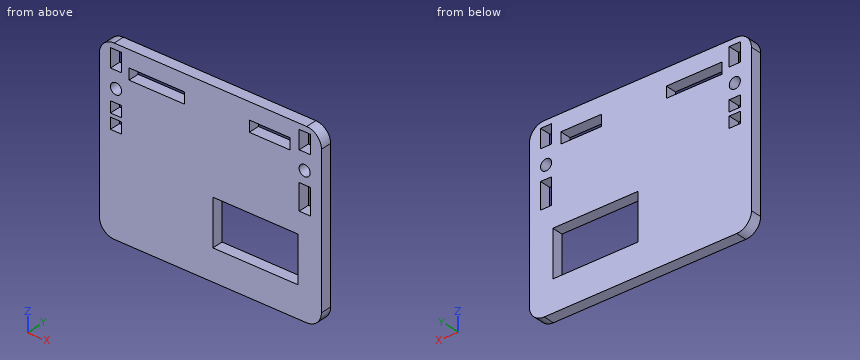
```python
from build123d import *

# Parameters (mm, degrees)
CROQUIS1_R                 = 1.5
CROQUIS1_W                 = 15
CROQUIS1_H                 = 3
CROQUIS1_W_2               = 3.003677296
CROQUIS1_H_2               = 7.000000001
CROQUIS1_W_3               = 23
CROQUIS1_H_3               = 12.400000001
SALIENTE_EXTRUIR1_DEPTH    = 3
S_LIDO_MOVER_COPIAR2_ANGLE = 90


with BuildPart() as part:
    # Croquis1 → Saliente-Extruir1 (new body)
    with BuildSketch(Plane(origin=(0, 0, 0), x_dir=(-1, 0, 0), z_dir=(0, 0, 1))):
        with BuildLine():
            Line((41781.908830987, 309.199124202), (41833.908830987, 309.199124202))
            ThreePointArc((41833.908830987, 309.199124202), (41836.737258112, 310.370697077), (41837.908830987, 313.199124202))
            Line((41837.908830987, 313.199124202), (41837.908830987, 353.199124202))
            ThreePointArc((41837.908830987, 353.199124202), (41836.737258112, 356.027551327), (41833.908830987, 357.199124202))
            Line((41833.908830987, 357.199124202), (41781.908830987, 357.199124202))
            ThreePointArc((41781.908830987, 357.199124202), (41779.080403863, 356.027551327), (41777.908830987, 353.199124202))
            Line((41777.908830987, 353.199124202), (41777.908830987, 313.199124202))
            ThreePointArc((41777.908830987, 313.199124202), (41779.080403863, 310.370697077), (41781.908830987, 309.199124202))
        make_face()
        with Locations(Location((41833.408830987, 320.199124198, 0), (0, 0, 180))):
            Circle(CROQUIS1_R, mode=Mode.SUBTRACT)
        with Locations(Location((41782.429915347, 320.197748539, 0), (0, 0, 180))):
            Circle(CROQUIS1_R, mode=Mode.SUBTRACT)
        Polygon((41786.408830987, 313.699124203), (41796.408830987, 313.699124203), (41797.408830987, 313.699124203), (41797.408830987, 316.699124203), (41796.408830987, 316.699124203), (41786.408830987, 316.699124203), align=None, mode=Mode.SUBTRACT)
        Polygon((41780.927290538, 315.695638799), (41783.429912384, 315.695638799), (41783.927165547, 315.695638799), (41783.929915347, 310.699124202), (41780.929915347, 310.699124202), align=None, mode=Mode.SUBTRACT)
        Polygon((41831.908830987, 310.699124202), (41834.408830987, 310.699124202), (41834.908830987, 310.699124202), (41834.908830987, 315.699124202), (41834.408830987, 315.699124202), (41831.908830987, 315.699124202), align=None, mode=Mode.SUBTRACT)
        Polygon((41831.908830987, 323.699124202), (41834.408830987, 323.699124202), (41834.908830987, 323.699124202), (41834.908830987, 326.699124202), (41834.408830987, 326.699124202), (41831.908830987, 326.699124202), align=None, mode=Mode.SUBTRACT)
        Polygon((41831.908830987, 327.699124202), (41834.408830987, 327.699124202), (41834.908830987, 327.699124202), (41834.908830987, 330.699124202), (41834.408830987, 330.699124202), (41831.908830987, 330.699124202), align=None, mode=Mode.SUBTRACT)
        with Locations((41822.408830987, 315.199124203)):
            Rectangle(CROQUIS1_W, CROQUIS1_H, mode=Mode.SUBTRACT)
        with Locations((41782.421247435, 327.199124203)):
            Rectangle(CROQUIS1_W_2, CROQUIS1_H_2, mode=Mode.SUBTRACT)
        with Locations((41795.738219532, 342.622009866)):
            Rectangle(CROQUIS1_W_3, CROQUIS1_H_3, mode=Mode.SUBTRACT)
    extrude(amount=SALIENTE_EXTRUIR1_DEPTH)


with BuildPart() as part_1:
    # Sólido-Mover/Copiar2: moved
    add(part.part.rotate(Axis((0, -333.199124202, 1.5), (1, 0, 0)), S_LIDO_MOVER_COPIAR2_ANGLE))


solid = part_1.part
```
Geometry check sheet. Reference: the model listing, model coordinates, mm. Coordinates: 2 decimals unless noted, no trailing zeros. Write each loop counter-clockwise with the first axis right and the second up, starting at its lowest first coordinate (ties: lowest second). Pieces come first, ordered by that corner, then holes. Notation, with made-up numbers: (-15, -19.5) -> (17, -19.5) arc R20 ccw to (17, 4.5) -> close; hole circle Ø1 at (72, 24.25). An arc over 180 degrees is marked (long way). Use CSV: the item, a comma, the result in double quotes. Start each with the question number.
Item 1: Thickness scan on line 1 (X direction, y = -332.4, z = 5.5); line 2 (Z direction, x = -41795.5, y = -334.05); line 3 (Z direction, x = -41833, y = -332.3). Record the ranges inside material, lowest first.
Item 2: Cross-section at A-A, the plane z = -3. Record the cut outline in (x, y), plus the area to 3 significant figures.
Item 3: Cross-section at C-C, the plane y = -333.25. State how many separate pieces and enclosed holes the cut face has, plus the area to 3 significant figures.
Item 4: Cross-section at B-B, the plane x = -41800. Record the cut outline in (y, z).
Answers:
1,line 1,"-41837.91 to -41834.91, -41831.91 to -41783.92, -41780.92 to -41777.91"
1,line 2,"-22.5 to -14.12, -1.72 to 18, 21 to 25.5"
1,line 3,"-22.5 to 4, 7 to 8, 11 to 13.06, 15.94 to 19, 24 to 25.5"
2,outline,"(-41837.91, -334.7) -> (-41807.24, -334.7) -> (-41807.24, -331.7) -> (-41837.91, -331.7) -> close; (-41784.24, -334.7) -> (-41777.91, -334.7) -> (-41777.91, -331.7) -> (-41784.24, -331.7) -> close"
2,area,"111 mm^2"
3,separate pieces,"1"
3,enclosed holes,"10"
3,area,"2,420 mm^2"
4,outline,"(-334.7, -22.5) -> (-331.7, -22.5) -> (-331.7, -14.12) -> (-334.7, -14.12) -> close; (-334.7, -1.72) -> (-331.7, -1.72) -> (-331.7, 25.5) -> (-334.7, 25.5) -> close"
